Geometry: final body of the model. Coordinates: model frame, mm. Face numbers are marked on the shaded views. A direction names the side the tool comes from. Coordinates: 2 decimals unless noted, no trailing zeros. Loops run counter-clockwise (first coordinate to the right, second up) from the corner with the lowest first, then second, coordinate; pieces in that order, holes last. Notation, with made-up numbers: M -17,4.25 L 39,4.25 A7 ccw 39,8.25 Z; hole C 71.5,-36 d2. An arc over 180 degrees is marked long. Write each question's results on one line, items separated by ' | '. Start each with the question number.
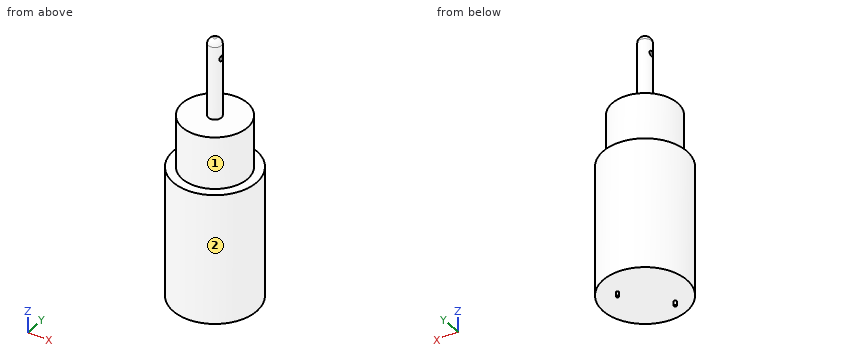
Autodesk Inventor part; units mm, degrees
ref_plane "YZ Plane" through (0, 0, 0) normal (1, 0, 0) x (0, 1, 0)
ref_plane "XZ Plane" through (0, 0, 0) normal (0, 1, 0) x (-1, 0, 0)
ref_plane "XY Plane" through (0, 0, 0) normal (0, 0, 1) x (1, 0, 0)
sketch "Sketch1" plane through (0, 0, 0) normal (0, 0, 1) x (1, 0, 0)
  circle A0 centre (0, 0) radius 16
  dimension "d0" = 32
extrude "Extrusion1" add sketch "Sketch1" along normal blind 50
sketch "Sketch2" plane through (0, 0, 50) normal (0, 0, 1) x (1, 0, 0)
  circle A0 centre (0, 0) radius 12.5
  dimension "d3" = 25
extrude "Extrusion2" add sketch "Sketch2" along normal blind 20
thread "Thread1"
sketch "Sketch3" plane through (0, 0, 70) normal (0, 0, 1) x (1, 0, 0)
  circle A0 centre (0, 0) radius 2.5
  dimension "d8" = 5
extrude "Extrusion3" add sketch "Sketch3" along normal blind 30
sketch "Sketch4" plane through (0, 0, 0) normal (1, 0, 0) x (0, 1, 0)
  line L0 (2.5, 100) -> (-2.5, 100)
  line L1 (0, 100) -> (0, 93)
  circle A0 centre (0, 93) radius 1
  point P0 (0, 0)
  dimension "d11" = 7
  dimension "d12" = 2
extrude "Extrusion4" cut sketch "Sketch4" along normal through all both and the other way through all
fillet "Fillet1" radius 2 1 edges at (-2.5, 0, 100)
sketch "Sketch5" plane through (0, 0, 0) normal (0, 0, 1) x (1, 0, 0)
  circle A0 centre (6.35, 6.35) radius 0.5
  circle A1 centre (-7.9375, -6.35) radius 0.5
  point P0 (0, 0)
  dimension "d16" = 1
  dimension "d17" = 1
extrude "Extrusion5" add sketch "Sketch5" against normal blind 1.7 contours A0
sketch "Sketch6" plane through (0, 0, 0) normal (0, 0, -1) x (-1, 0, 0)
  circle A0 centre (6.35, -7.9375) radius 0.5
  point P0 (0, 0)
  dimension "d20" = 1
extrude "Extrusion6" add sketch "Sketch6" along normal blind 1.7
sketch "Sketch7" plane through (0, 0, 0) normal (0, 0, -1) x (-1, 0, 0)
  circle A0 centre (-6.35, 6.35) radius 0.5
  line L0 (-6.35, 6.35) -> (-42.8625, 12.7) construction
  line L1 (-42.8625, 12.7) -> (-28.575, -14.2875) construction
  line L2 (-28.575, -14.2875) -> (-46.0375, -6.35) construction
  line L3 (-46.0375, -6.35) -> (-31.75, -22.225) construction
  spline S0 degree 4 poles (-6.35, 6.35) (-42.8625, 12.7) (-28.575, -14.2875) (-46.0375, -6.35) (-31.75, -22.225) knots 1 1 1 1 1 2 2 2 2 2
  line L4 (6.35, -7.9375) -> (-22.6919, -25.4) construction
  line L5 (-22.6919, -25.4) -> (-14.2875, -33.3375) construction
  spline S1 degree 2 poles (6.35, -7.9375) (-22.6919, -25.4) (-14.2875, -33.3375) knots 1 1 1 2 2 2
  point P0 (0, 0)
properties part number "dc motor"
Item 1: Contact query for flat-ended pins moving along their axis: P1, Ø2, axis at x = 1, y = -11, coming from the +Z side; P2, Ø5, axis at x = -7, y = 5, coming from the -Z side; P3, Ø2, axis at x = 7.5, z = 47, coming from the +Y side. Output: stop coordinate, or through.
Item 2: Section B-B, the plane x = -11.5. Return loops of the section in (y, z), plus the area to 3 significant figures.
Item 3: Section D-D, the plane z = 78. Return loops of the section in (x, y).
Item 4: Section A-A, the plane z = 93. Return loops of the section in (x, y), plus the area to 3 significant figures.
Item 5: Set-up query: the marked faces 1 and 2. Return all of +Z, -Z, +X, -X, +Y, -Y with unobstructed straight access to the full face (end or side cutting, diameter ignored); none if empty.
Item 6: Ray query, L1, parallel to Z at x = 0, y = 0; L2, parallel to Y at x = -0.3, z = 93; L3, parallel to Y at x = 0, z = 61.5. Return the intervals inside material, ascending. Write a range as [from, to].
Item 7: Section C-C, the plane y = 9. Return loops of the section in (x, z), plus the area to 3 significant figures.
Solutions:
1) P1: stops at z = 70 | P2: stops at z = 0 | P3: stops at y = 14.62
2) outline: M -11.12,0 L 11.12,0 L 11.12,50 L 4.9,50 L 4.9,70 L -4.9,70 L -4.9,50 L -11.12,50 Z | area: 1,310 mm²
3) outline: C 0,0 d5
4) outline: M -2.29,-1 A2.5 ccw 2.29,-1 Z; M -2.29,1 L 2.29,1 A2.5 ccw Z | area: 9.91 mm²
5) face 1: +Z | face 2: +Z, -Z
6) L1: z = [0, 92], [94, 100] | L2: y = [-2.48, -1], [1, 2.48] | L3: y = [-12.5, 12.5]
7) outline: M -13.23,0 L 13.23,0 L 13.23,50 L 8.67,50 L 8.67,70 L -8.67,70 L -8.67,50 L -13.23,50 Z | area: 1,670 mm²
